Source: CAD feature listing. Evaluate the final solid. Frame: model axes, mm. Face numbers are marked on the shaded views. A direction names the side the tool comes from. Round coordinates to 2 decimals unless told otherwise and drop trailing zeros. Loops run counter-clockwise (first coordinate to the right, second up) from the corner with the lowest first, then second, coordinate; pieces in that order, holes last. Notation, with made-up numbers: (34, 28.25) -> (45, 28.25) arc R22 ccw to (45, 65.25) -> close; hole circle Ø7 at (46.25, 53). An arc over 180 degrees is marked (long way). Write item = value, one per line.
from build123d import *

# Parameters (mm, degrees)
SKETCH1_W           = 30
SKETCH1_H           = 30
SKETCH1_R           = 2
BOSS_EXTRUDE1_DEPTH = 10


with BuildPart() as part:
    # Sketch1 → Boss-Extrude1 (new body)
    with BuildSketch(Plane(origin=(0, 0, 0), x_dir=(0, 0, -1), z_dir=(1, 0, 0))):
        Rectangle(SKETCH1_W, SKETCH1_H)
        with Locations((8.414570696, 8.414570696)):
            Circle(SKETCH1_R, mode=Mode.SUBTRACT)
        with Locations((8.414570696, -8.414570696)):
            Circle(SKETCH1_R, mode=Mode.SUBTRACT)
        with Locations((-8.414570696, -8.414570696)):
            Circle(SKETCH1_R, mode=Mode.SUBTRACT)
        with Locations((-8.414570696, 8.414570696)):
            Circle(SKETCH1_R, mode=Mode.SUBTRACT)
        with BuildLine():
            ThreePointArc((-1.274653828, 7.644459276), (0, 6.470984275), (1.274653828, 7.644459276))
            ThreePointArc((1.274653828, 7.644459276), (2.394881706, 7.370688001), (3.462083815, 6.933720189))
            ThreePointArc((3.462083815, 6.933720189), (3.803549125, 5.235136249), (5.524517033, 5.435274745))
            ThreePointArc((5.524517033, 5.435274745), (6.269881706, 4.555335705), (6.876423113, 3.574535658))
            ThreePointArc((6.876423113, 3.574535658), (6.154271761, 1.999644111), (7.664202503, 1.15))
            ThreePointArc((7.664202503, 1.15), (7.75, 0), (7.664202503, -1.15))
            ThreePointArc((7.664202503, -1.15), (6.154271761, -1.999644111), (6.876423113, -3.574535658))
            ThreePointArc((6.876423113, -3.574535658), (6.269881706, -4.555335705), (5.524517033, -5.435274745))
            ThreePointArc((5.524517033, -5.435274745), (3.803549125, -5.235136249), (3.462083815, -6.933720189))
            ThreePointArc((3.462083815, -6.933720189), (2.394881706, -7.370688001), (1.274653828, -7.644459276))
            ThreePointArc((1.274653828, -7.644459276), (0, -6.470984275), (-1.274653828, -7.644459276))
            ThreePointArc((-1.274653828, -7.644459276), (-2.394881706, -7.370688001), (-3.462083815, -6.933720189))
            ThreePointArc((-3.462083815, -6.933720189), (-3.803549125, -5.235136249), (-5.524517033, -5.435274745))
            ThreePointArc((-5.524517033, -5.435274745), (-6.269881706, -4.555335705), (-6.876423113, -3.574535658))
            ThreePointArc((-6.876423113, -3.574535658), (-6.154271761, -1.999644111), (-7.664202503, -1.15))
            ThreePointArc((-7.664202503, -1.15), (-7.75, 0), (-7.664202503, 1.15))
            ThreePointArc((-7.664202503, 1.15), (-6.154271761, 1.999644111), (-6.876423113, 3.574535658))
            ThreePointArc((-6.876423113, 3.574535658), (-6.269881706, 4.555335705), (-5.524517033, 5.435274745))
            ThreePointArc((-5.524517033, 5.435274745), (-3.803549125, 5.235136249), (-3.462083815, 6.933720189))
            ThreePointArc((-3.462083815, 6.933720189), (-2.394881706, 7.370688001), (-1.274653828, 7.644459276))
        make_face(mode=Mode.SUBTRACT)
    extrude(amount=BOSS_EXTRUDE1_DEPTH)


solid = part.part
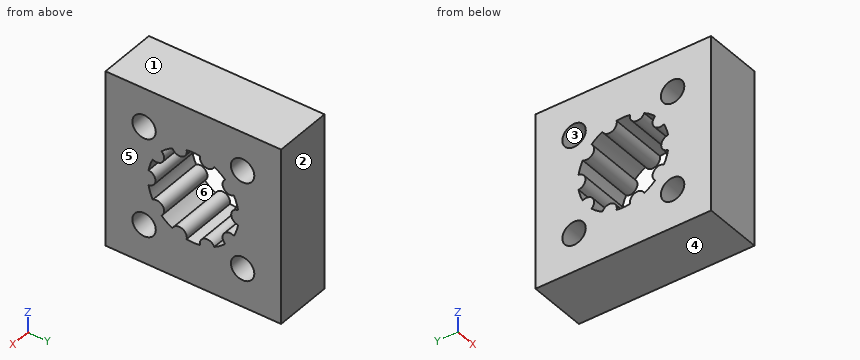
1. Section query B-B (y = 8). Return the cut outline in (x, z), then the cut area to 3 significant figures.
Evaluation:
outline = (0, -15) -> (10, -15) -> (10, -10.37) -> (0, -10.37) -> close; (0, -6.46) -> (10, -6.46) -> (10, 6.46) -> (0, 6.46) -> close; (0, 10.37) -> (10, 10.37) -> (10, 15) -> (0, 15) -> close
area = 222 mm²
2. Contact query for a flat-ended pin moving along its axis: pin 1 Ø6 at (y, z) = (-1, 4.5) entering from +X. Output: stop coordinate, or through.
Evaluation:
pin_1 = 10
3. Section query D-D (z = 2.75). Return the cut outline in (x, y).
Evaluation:
outline = (0, -15) -> (10, -15) -> (10, -7.25) -> (0, -7.25) -> close; (0, 7.25) -> (10, 7.25) -> (10, 15) -> (0, 15) -> close
4. Line query: probe 1 along Z at (x, y) = (9.5, -8.5); probe 2 along Z at (x, y) = (9, -2.5); probe 3 along Y at (x, z) = (7.75, -9.75). Output: solid intervals per line, ascending. Write a range as from..to.
Evaluation:
probe_1 = -15..-10.41, -6.42..6.42, 10.41..15
probe_2 = -15..-6.1, 6.1..15
probe_3 = -15..-9.9, -6.93..6.93, 9.9..15
5. Set-up query: the marked faces 5 and 6. Return all of +Z, -Z, +X, -X, +Y, -Y with unobstructed straight access to the full face (end or side cutting, diameter ignored); none if empty.
Evaluation:
face_5 = +Z, -Z, +X, +Y, -Y
face_6 = +X, -X
6. Section query A-A (z = -8.5). Return the cut outline in (x, y).
Evaluation:
outline = (0, -15) -> (10, -15) -> (10, -10.41) -> (0, -10.41) -> close; (0, -6.42) -> (10, -6.42) -> (10, 6.42) -> (0, 6.42) -> close; (0, 10.41) -> (10, 10.41) -> (10, 15) -> (0, 15) -> close
7. Section query C-C (y = -0.75). Return the cut outline in (x, z), then the cut area to 3 significant figures.
Evaluation:
outline = (0, -15) -> (10, -15) -> (10, -7.71) -> (0, -7.71) -> close; (0, 7.71) -> (10, 7.71) -> (10, 15) -> (0, 15) -> close
area = 146 mm²
8. Mould query, pull axis Z, two halves, no side actions, for the marked faces 1, 2, 3 and 4. Classes: released by +Z, released by -Z, zero draft, split by the parting line, or undercut.
Evaluation:
face_1 = released by +Z
face_2 = zero draft
face_3 = undercut
face_4 = released by -Z
